from build123d import *

# Parameters (mm, degrees)
SKETCH1_R               = 33.85
BOSS_EXTRUDE1_DEPTH     = 12.5
SKETCH2_R               = 2.5
CUT_EXTRUDE1_DEPTH      = 34.85
CUT_EXTRUDE1_DEPTH_BACK = 34.85
SKETCH3_R               = 2.5
CUT_EXTRUDE2_DEPTH      = 34.8500001
CUT_EXTRUDE2_DEPTH_BACK = 34.8500001
SKETCH4_R               = 42.35
BOSS_EXTRUDE2_DEPTH     = 2
SKETCH5_R               = 42.35
SKETCH5_R_2             = 33.85
BOSS_EXTRUDE3_DEPTH     = 120
SKETCH6_R               = 2.5
CUT_EXTRUDE3_DEPTH      = 43.35
CUT_EXTRUDE3_DEPTH_BACK = 43.35
SKETCH7_R               = 2.5
CUT_EXTRUDE4_DEPTH      = 43.3500001
CUT_EXTRUDE4_DEPTH_BACK = 43.3500001
CUT_EXTRUDE5_DEPTH      = 120


with BuildPart() as part:
    # Sketch1 → Boss-Extrude1 (new body)
    with BuildSketch(Plane(origin=(0, 0, 0), x_dir=(1, 0, 0), z_dir=(0, 1, 0))):
        Circle(SKETCH1_R)
    extrude(amount=BOSS_EXTRUDE1_DEPTH)

    # Sketch2 → Cut-Extrude1 (cut, two sides)
    with BuildSketch(Plane(origin=(0, 0, 0), x_dir=(0, 0, -1), z_dir=(1, 0, 0))) as cut_extrude1_sk:
        with Locations((0, 5)):
            Circle(SKETCH2_R)
    extrude(amount=CUT_EXTRUDE1_DEPTH, mode=Mode.SUBTRACT)
    extrude(cut_extrude1_sk.sketch, amount=-CUT_EXTRUDE1_DEPTH_BACK, mode=Mode.SUBTRACT)

    # Sketch3 → Cut-Extrude2 (cut, two sides)
    with BuildSketch(Plane.XY) as cut_extrude2_sk:
        with Locations((0, 5)):
            Circle(SKETCH3_R)
    extrude(amount=CUT_EXTRUDE2_DEPTH, mode=Mode.SUBTRACT)
    extrude(cut_extrude2_sk.sketch, amount=-CUT_EXTRUDE2_DEPTH_BACK, mode=Mode.SUBTRACT)

    # Sketch4 → Boss-Extrude2 (add)
    with BuildSketch(Plane(origin=(0, 12.5, 0), x_dir=(1, 0, 0), z_dir=(0, 1, 0))):
        Circle(SKETCH4_R)
    extrude(amount=BOSS_EXTRUDE2_DEPTH)

    # Sketch5 → Boss-Extrude3 (add)
    with BuildSketch(Plane(origin=(0, 14.5, 0), x_dir=(1, 0, 0), z_dir=(0, 1, 0))):
        Circle(SKETCH5_R)
        Circle(SKETCH5_R_2, mode=Mode.SUBTRACT)
    extrude(amount=BOSS_EXTRUDE3_DEPTH)

    # Sketch6 → Cut-Extrude3 (cut, two sides)
    with BuildSketch(Plane(origin=(0, 0, 0), x_dir=(0, 0, -1), z_dir=(1, 0, 0))) as cut_extrude3_sk:
        with Locations((0, 127)):
            Circle(SKETCH6_R)
    extrude(amount=CUT_EXTRUDE3_DEPTH, mode=Mode.SUBTRACT)
    extrude(cut_extrude3_sk.sketch, amount=-CUT_EXTRUDE3_DEPTH_BACK, mode=Mode.SUBTRACT)

    # Sketch7 → Cut-Extrude4 (cut, two sides)
    with BuildSketch(Plane.XY) as cut_extrude4_sk:
        with Locations((0, 127)):
            Circle(SKETCH7_R)
    extrude(amount=CUT_EXTRUDE4_DEPTH, mode=Mode.SUBTRACT)
    extrude(cut_extrude4_sk.sketch, amount=-CUT_EXTRUDE4_DEPTH_BACK, mode=Mode.SUBTRACT)

    # Sketch9 → Cut-Extrude5 (cut)
    with BuildSketch(Plane(origin=(0, 134.5, 0), x_dir=(1, 0, 0), z_dir=(0, 1, 0))):
        Polygon((24.112341238, 26.587214973), (-26.587214973, -24.112341238), (-24.112341238, -26.587214973), (26.587214973, 24.112341238), align=None)
    extrude(amount=-CUT_EXTRUDE5_DEPTH, mode=Mode.SUBTRACT)


solid = part.part
Can you work these out from the model? Positions are in its coordinate system, mm. A direction names the side the tool comes from. Round coordinates to 2 decimals unless told otherwise and drop trailing zeros. Write each loop counter-clockwise with the first axis right and the second up, starting at its lowest first coordinate (ties: lowest second). Pieces come first, ordered by that corner, then holes. Notation, with made-up numbers: (67.25, 34.25) - (115.25, 34.25) arc R24 ccw to (115.25, 68.25) - close; hole circle Ø6 at (59.5, 16). An arc over 180 degrees is marked (long way). Write each question's results on one line, items separated by ' | '. Start each with the question number.
1) Suppose I cut it at B-B (y = 76). List the corners of the cut face in (x, z) for me.
2) Please list where these lines run through material, in increasing order: line 1 (X direction, y = 31.5, z = 0); line 2 (Y direction, x = -20, z = 36); line 3 (Y direction, x = 0, z = 16.5).
3) Suppose I cut it at C-C (x = -8). List the corners of the cut face in (y, z) for me, and give its area (3 significant figures).
4) Suppose I cut it at A-A (y = 5). List the corners of the cut face in (x, z) for me, and give its area (3 significant figures).
5) We'd pull the mould along X, two halves only. Please class faces 1 (the flat face through (0, 0, 0)), 2 (the cylindrical face through (40.4, 72.6, -12.7)), 3 (the cylindrical face through (23.42, 73.66, 24.44)), 4 (the cylindrical face through (1.34, 129.11, -37.99)): released by +X, released by -X, zero draft, split by the parting line, or undercut.
6) For pin 1 Ø4 at (x, y) = (0, 127) entering from -Z; pin 2 Ø1.5 at (x, y) = (21.5, 32.5) entering from -Z; pin 3 Ø2 at (x, y) = (-14.5, 32.5) entering from +Z; pin 4 Ø8 at (y, z) = (127, 0) entering from -X, each with a flat end and sliding along its axis, tell me the tip position at first contact or that it passes through.
7) Which directions (+Z, -Z, +X, -X, +Y, -Y) give clear straight access to the entire face, cutting with the end or side of a thin tool? Please do faces 5 (the flat face through (0, 14.5, 0)), 6 (the cylindrical face through (32.287, 6.162, -10.168)), 7 (the cylindrical face through (2.385, 5.751, 16.689)).
8) Suppose I cut it at D-D (z = -14). List the corners of the cut face in (x, y) for me, and give its area (3 significant figures).
Here are the results:
1) outline: circle Ø84.7 at (0, 0); hole (-26.59, 24.11) - (-25.14, 22.67) arc R33.85 ccw to (22.67, -25.14) - (24.11, -26.59) - (26.59, -24.11) - (25.14, -22.67) arc R33.85 ccw to (-22.67, 25.14) - (-24.11, 26.59) - close
2) line 1: x = -42.35 to -33.85, 33.85 to 42.35 | line 2: y = 12.5 to 134.5 | line 3: y = 0 to 2.5, 7.5 to 14.5
3) outline: (0, -32.89) - (12.5, -32.89) - (12.5, -41.59) - (134.5, -41.59) - (134.5, -32.89) - (14.5, -32.89) - (14.5, 32.89) - (134.5, 32.89) - (134.5, 41.59) - (12.5, 41.59) - (12.5, 32.89) - (0, 32.89) - close; hole circle Ø5 at (5, 0) | area: 3,060 mm2
4) outline: (-33.76, -2.5) arc R33.85 ccw to (-2.5, -33.76) - (-2.5, -2.5) - close; (-33.76, 2.5) - (-2.5, 2.5) - (-2.5, 33.76) arc R33.85 ccw to start; (2.5, -33.76) arc R33.85 ccw to (33.76, -2.5) - (2.5, -2.5) - close; (2.5, 2.5) - (33.76, 2.5) arc R33.85 ccw to (2.5, 33.76) - close | area: 2,950 mm2
5) face 1: zero draft | face 2: split by the parting line | face 3: undercut | face 4: undercut
6) pin 1: passes through | pin 2: stops at z = -36.92 | pin 3: stops at z = 40.14 | pin 4: stops at x = -42.35
7) face 5: +Y | face 6: -Y | face 7: +Z, -Z
8) outline: (-39.97, 12.5) - (-30.82, 12.5) - (-30.82, 0) - (30.82, 0) - (30.82, 12.5) - (39.97, 12.5) - (39.97, 134.5) - (30.82, 134.5) - (30.82, 14.5) - (-30.82, 14.5) - (-30.82, 134.5) - (-39.97, 134.5) - close; hole circle Ø5 at (0, 5) | area: 3,110 mm2
